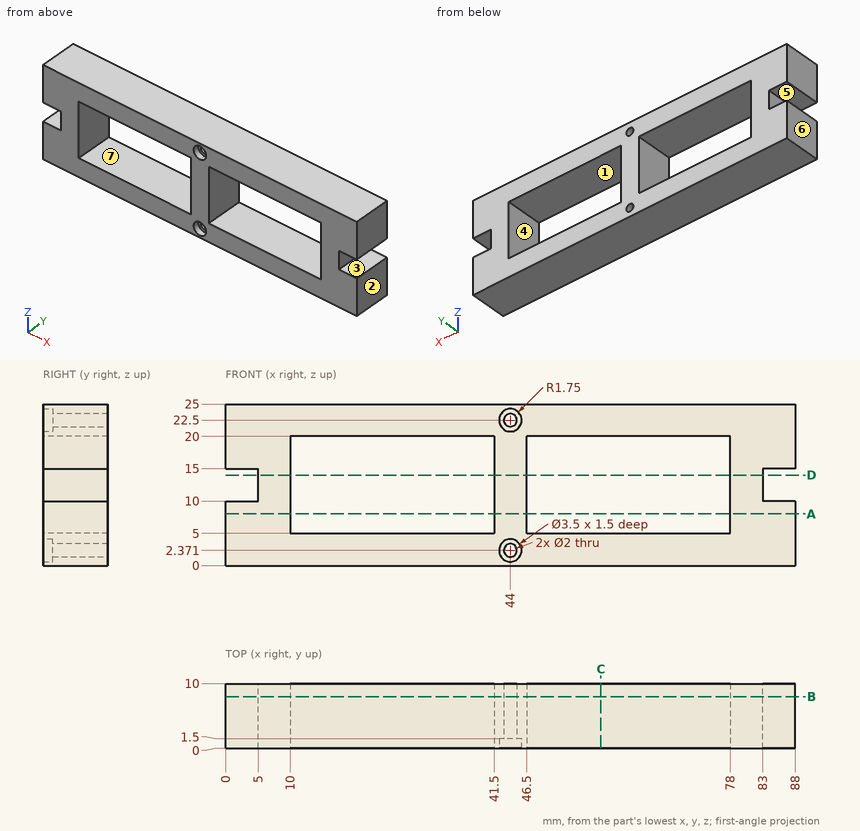
Answer from the drawing. Dimensions are ordinates in mm from the lowest x, y and z of the part. A direction names the side the tool comes from. Coordinates: 2 decimals unless noted, no trailing zeros. Loops run counter-clockwise (first coordinate to the right, second up) from the corner with the lowest first, then second, coordinate; pieces in that order, holes last.
1) Section D-D (z = 14) is taken. Give the vertices of the cut face in (x, y).
Results:
outline: (5, 0) - (10, 0) - (10, 10) - (5, 10) - close; (41.5, 0) - (46.5, 0) - (46.5, 10) - (41.5, 10) - close; (78, 0) - (83, 0) - (83, 10) - (78, 10) - close
2) For the marked faces 1, 2 and 3, determine the directions among +Z, -Z, +X, -X, +Y, -Y from which every point of the face is accessible in a straight line to the end or side of a thin tool.
Results:
face 1: +Y, -Y
face 2: +Z, -Z, +X, +Y, -Y
face 3: +X, +Y, -Y
3) Section A-A (z = 8) is taken. Give the vertices of the cut face in (x, y).
Results:
outline: (0, 0) - (10, 0) - (10, 10) - (0, 10) - close; (41.5, 0) - (46.5, 0) - (46.5, 10) - (41.5, 10) - close; (78, 0) - (88, 0) - (88, 10) - (78, 10) - close
4) For a pull along X with two mould halves and no side action, classify the marked faces 4, 5, 6 and 7 as +X half, -X half, draft (parallel to the pull), parting line (faces both ways), or undercut.
Results:
face 4: undercut
face 5: draft
face 6: -X half
face 7: undercut
5) Section C-C (x = 58) is taken. Give the vertices of the cut face in (y, z).
Results:
outline: (0, 0) - (10, 0) - (10, 5) - (0, 5) - close; (0, 20) - (10, 20) - (10, 25) - (0, 25) - close
6) Consider probe 1 along X at (y, z) = (1.5, 12.75); probe 2 along X at (y, z) = (4.75, 18.75); probe 3 along Z at (x, y) = (57.5, 7.5). Determine where each line is inside the solid, lowest interval first.
Results:
probe 1: x = 5 to 10, 41.5 to 46.5, 78 to 83
probe 2: x = 0 to 10, 41.5 to 46.5, 78 to 88
probe 3: z = 0 to 5, 20 to 25
7) A flat-ended cylindrical pin translates along its axis: pin 1 (1.5 mm diameter, centred on y = 6, z = 12.5, fed in from -X). Find the tip coordinate at first contact, or state that the pin passes through.
Results:
pin 1: stops at x = 5
8) Section B-B (y = 8) is taken. Give the vertices of the cut face in (x, z), plus the area to 3 significant figures.
Results:
outline: (0, 0) - (88, 0) - (88, 10) - (83, 10) - (83, 15) - (88, 15) - (88, 25) - (0, 25) - (0, 15) - (5, 15) - (5, 10) - (0, 10) - close; hole (10, 5) - (41.5, 5) - (41.5, 20) - (10, 20) - close; hole circle Ø2 at (44, 2.37); hole circle Ø2 at (44, 22.5); hole (46.5, 5) - (78, 5) - (78, 20) - (46.5, 20) - close
area: 1,200 mm2
